from build123d import *

# Parameters (mm, degrees)
BASPROSKE_W         = 12.5
BASPROSKE_H         = 14.375
TOOTHCUT_DEPTH      = 24.864853865
TEETHCUTS_COUNT     = 21
TEETHCUTS_ANGLE     = 342.857142857
BORSKE_R            = 4
BORE_DEPTH          = 50.0000508
SKETCH1_R           = 7.5
BOSS_EXTRUDE1_DEPTH = 100
SKETCH2_W           = 3
SKETCH2_H           = 2
CUT_EXTRUDE1_DEPTH  = 16.8


with BuildPart() as part:
    # BasProSke → Base-Revolve (revolve)
    with BuildSketch(Plane(origin=(0, 0, 0), x_dir=(1, 0, 0), z_dir=(0, 1, 0)), mode=Mode.PRIVATE) as base_revolve_sk:
        with Locations((6.25, 7.1875)):
            Rectangle(BASPROSKE_W, BASPROSKE_H)
    revolve(base_revolve_sk.sketch.rotate(Axis((-10, 0, 0), (1, 0, 0)), 180), axis=Axis((-10, 0, 0), (1, 0, 0)))

    # TooCutSke → ToothCut (cut, through all)
    with BuildSketch(Plane(origin=(0, 0, 0), x_dir=(0, 0, -1), z_dir=(1, 0, 0))):
        with BuildLine():
            ThreePointArc((0.615260942, 11.545117419), (0, 11.5615), (-0.615260942, 11.545117419))
            ThreePointArc((-0.615260942, 11.545117419), (-1.023565158, 13.002884474), (-1.830858013, 14.283538746))
            ThreePointArc((-1.830858013, 14.283538746), (0, 14.4004), (1.830858013, 14.283538746))
            ThreePointArc((1.830858013, 14.283538746), (1.023565158, 13.002884474), (0.615260942, 11.545117419))
        make_face()
    toothcut = extrude(amount=TOOTHCUT_DEPTH, mode=Mode.SUBTRACT)

    # TeethCuts: ToothCut ×21 about axis
    teethcuts_axis = Axis((-10, 0, 0), (1, 0, 0))
    for i in range(1, TEETHCUTS_COUNT):
        add(toothcut.rotate(teethcuts_axis, i * TEETHCUTS_ANGLE / (TEETHCUTS_COUNT - 1)), mode=Mode.SUBTRACT)

    # BorSke → Bore (cut, symmetric)
    with BuildSketch(Plane(origin=(0, 0, 0), x_dir=(0, 0, -1), z_dir=(1, 0, 0))):
        with Locations(Location((0, 0, 0), (0, 0, 180))):
            Circle(BORSKE_R)
    extrude(amount=BORE_DEPTH, both=True, mode=Mode.SUBTRACT)

    # Sketch1 → Boss-Extrude1 (add)
    with BuildSketch(Plane.ZY):
        Circle(SKETCH1_R)
    extrude(amount=-BOSS_EXTRUDE1_DEPTH)

    # Sketch2 → Cut-Extrude1 (cut)
    with BuildSketch(Plane(origin=(100, 0, 0), x_dir=(0, 0, -1), z_dir=(1, 0, 0))):
        with Locations((-7.5, 0)):
            Rectangle(SKETCH2_W, SKETCH2_H)
    extrude(amount=-CUT_EXTRUDE1_DEPTH, mode=Mode.SUBTRACT)


solid = part.part
Design review of the part built by this model. Coordinates are the model's own, in mm. A direction names the side the tool comes from. Round coordinates to 2 decimals unless told otherwise and drop trailing zeros. Write each loop counter-clockwise with the first axis right and the second up, starting at its lowest first coordinate (ties: lowest second). Pieces come first, ordered by that corner, then holes. Notation, with made-up numbers: (17.25, 85) - (26.25, 85) arc R27 ccw to (26.25, 110) - close; hole circle Ø6 at (60.5, 10). An arc over 180 degrees is marked (long way). Return JSON: item names as keys, results as strings. Group by question number.
Item 1: For probe 1 along X at (y, z) = (-8, -0.25); probe 2 along Z at (x, y) = (19.5, 3); probe 3 along Z at (x, y) = (56, 2.75), list the stretches that pass through material, from the lowest coordinate up. Write a range as [from, to].
Item 2: Insertion check: P1, Ø1.5, axis at x = 46, z = 3, coming from the -Y side; P2, Ø2, axis at x = 93, y = -0.5, coming from the +Z side; P3, Ø10, axis at x = 27.5, y = -9.5, coming from the +Z side; P4, Ø5, axis at y = -1.5, z = -1.5, coming from the -X side. Each pin has a flat end and moves straight along its axis. Give the tip position at first contact, or say it passes through.
Item 3: The part is to be moulded in two halves that separate along Z. For faces 1 (the face through (6.2, 2, 12.9)), 2 (the face through (6.162, -1.902, -12.869)), 3 (the face through (6.2, 2, -12.9)), say which applies: pulls with the +Z half, pulls with the -Z half, needs draft (parallel to the pull), parting line crosses it, or undercut.
Item 4: We need section A-A on x = 81.5. Write out the cut boundary in (y, z).
Item 5: Machinability: for faces 4 (the face through (6.162, 8.875, -9.511)), 5 (the face through (6.16, 12.69, -2.86)), 6 (the face through (6.162, 13.008, -1.026)), 7 (the face through (6.162, -0.037, 13.009)), which of the approach directions +Z, -Z, +X, -X, +Y, -Y give a long, thin tool a straight path to every point of the face, cutting with its end or side? Answer none if there is none.
Model answer:
{
 "1": {"probe 1": "x = [0, 12.5]", "probe 2": "z = [-6.87, 6.87]", "probe 3": "z = [-6.98, 6.98]"},
 "2": {"P1": "stops at y = -7.15", "P2": "stops at z = 7.43", "P3": "stops at z = 6", "P4": "stops at x = 0"},
 "3": {"face 1": "pulls with the +Z half", "face 2": "undercut", "face 3": "pulls with the -Z half"},
 "4": {"outline": "circle Ø15 at (0, 0)"},
 "5": {"face 4": "-Z, +X, -X", "face 5": "+X, -X", "face 6": "+X, -X, +Y", "face 7": "+Z, +X, -X"}
}
